Read the model definition and answer for the solid it produces. Units are mm, in the model's axes. Give positions to 0.01 mm unless a question says otherwise; leave off trailing zeros. Order: outer loops, then holes, each group sorted by start corner. A loop starts at its lowest first (then second) coordinate and runs counter-clockwise, first axis right, second up. Notation, with made-up numbers: (-1.5, 61.25) -> (38.5, 61.25) arc R17 cw to (38.5, 67.25) -> close; hole circle Ø7 at (-33.75, 81). An arc over 180 degrees is marked (long way). Use one line per item in the form item = value.
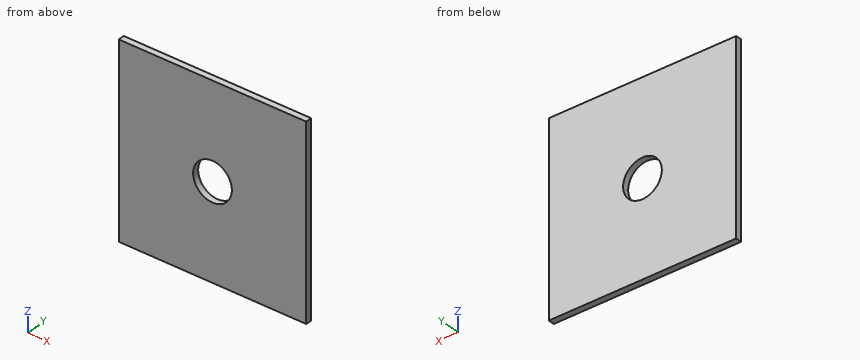
```python
from build123d import *

# Parameters (mm, degrees)
SKETCH2_W                = 30
SKETCH2_H                = 30
BOSS_EXTRUDE1_DEPTH      = 10
SKETCH3_W                = 30
SKETCH3_H                = 30
SKETCH3_W_2              = 25
SKETCH3_H_2              = 25
BOSS_EXTRUDE2_DEPTH      = 15
SKETCH4_W                = 30
SKETCH4_H                = 30
BOSS_EXTRUDE3_DEPTH      = 15
CUT_EXTRUDE1_START       = -40
SKETCH5_R                = 3.05
CUT_EXTRUDE1_DEPTH       = 40
BOSS_EXTRUDE4_DEPTH      = 10
BOSS_EXTRUDE4_DEPTH_BACK = 40
SKETCH6_W                = 7.5
SKETCH6_H                = 1.017843133
SKETCH6_H_2              = 1.2761833
SKETCH7_R                = 2.76
CUT_EXTRUDE2_DEPTH       = 10
SKETCH8_W                = 30
SKETCH8_H                = 30
BOSS_EXTRUDE5_DEPTH      = 1
SKETCH9_R                = 3.1
CUT_EXTRUDE3_DEPTH       = 1


with BuildPart() as part:
    # Sketch2 → Boss-Extrude1 (new body)
    with BuildSketch(Plane(origin=(0, 0, 0), x_dir=(1, 0, 0), z_dir=(0, 1, 0))):
        Rectangle(SKETCH2_W, SKETCH2_H)
    extrude(amount=BOSS_EXTRUDE1_DEPTH)


with BuildPart() as body_2:
    # Sketch3 → Boss-Extrude2 (new body)
    with BuildSketch(Plane(origin=(0, 10, 0), x_dir=(1, 0, 0), z_dir=(0, 1, 0))):
        Rectangle(SKETCH3_W, SKETCH3_H)
        Rectangle(SKETCH3_W_2, SKETCH3_H_2, mode=Mode.SUBTRACT)
    extrude(amount=BOSS_EXTRUDE2_DEPTH)


with BuildPart() as body_3:
    # Sketch4 → Boss-Extrude3 (new body)
    with BuildSketch(Plane(origin=(0, 25, 0), x_dir=(1, 0, 0), z_dir=(0, 1, 0))):
        Rectangle(SKETCH4_W, SKETCH4_H)
    extrude(amount=BOSS_EXTRUDE3_DEPTH)


with BuildPart() as cut_extrude1_tool:
    # Sketch5 → Cut-Extrude1 (new body)
    with BuildSketch(Plane(origin=(0, 40, 0), x_dir=(1, 0, 0), z_dir=(0, 1, 0)).offset(CUT_EXTRUDE1_START)):
        with Locations(Location((0, 0, 0), (0, 0, 270))):
            Circle(SKETCH5_R)
    extrude(amount=CUT_EXTRUDE1_DEPTH)


with BuildPart() as part_1:
    add(part.part)

    # Cut-Extrude1: cut by cut_extrude1_tool
    add(cut_extrude1_tool.part, mode=Mode.SUBTRACT)


with BuildPart() as body_3_1:
    add(body_3.part)

    # Cut-Extrude1: cut by cut_extrude1_tool
    add(cut_extrude1_tool.part, mode=Mode.SUBTRACT)

    # Sketch6 → Boss-Extrude4 (add, two sides: drawn at the far end of the back side and taken through both)
    with BuildSketch(Plane(origin=(0, 0, -15), x_dir=(-1, 0, 0), z_dir=(0, 0, -1)).offset(-BOSS_EXTRUDE4_DEPTH_BACK)):
        with Locations((-11.25, 25.508921566)):
            Rectangle(SKETCH6_W, SKETCH6_H)
        with Locations((11.25, 25.63809165)):
            Rectangle(SKETCH6_W, SKETCH6_H_2)
    extrude(amount=BOSS_EXTRUDE4_DEPTH + BOSS_EXTRUDE4_DEPTH_BACK)

    # Sketch7 → Cut-Extrude2 (cut)
    with BuildSketch(Plane(origin=(0, 26.2761833, 0), x_dir=(1, 0, 0), z_dir=(0, 1, 0))):
        with Locations(Location((-11.25, 20, 0), (0, 0, 270))):
            Circle(SKETCH7_R)
        with Locations(Location((11.25, 20, 0), (0, 0, 270))):
            Circle(SKETCH7_R)
        with Locations(Location((11.25, -20.5, 0), (0, 0, 270))):
            Circle(SKETCH7_R)
        with Locations(Location((-11.25, -20.5, 0), (0, 0, 270))):
            Circle(SKETCH7_R)
    extrude(amount=-CUT_EXTRUDE2_DEPTH, mode=Mode.SUBTRACT)


with BuildPart() as body_2_2:
    # Sketch8 → Boss-Extrude5 (new body)
    with BuildSketch(Plane(origin=(0, 40, 0), x_dir=(1, 0, 0), z_dir=(0, 1, 0))):
        Rectangle(SKETCH8_W, SKETCH8_H)
    extrude(amount=BOSS_EXTRUDE5_DEPTH)

    # Sketch9 → Cut-Extrude3 (cut)
    with BuildSketch(Plane(origin=(0, 41, 0), x_dir=(1, 0, 0), z_dir=(0, 1, 0))):
        with Locations(Location((0, 0, 0), (0, 0, 270))):
            Circle(SKETCH9_R)
    extrude(amount=-CUT_EXTRUDE3_DEPTH, mode=Mode.SUBTRACT)


solid = body_2_2.part
```
Item 1: The part is cut by section C-C on y = 40.8. Give the vertices of the cut face in (x, z).
Checks:
outline = (-15, -15) -> (15, -15) -> (15, 15) -> (-15, 15) -> close; hole circle Ø6.2 at (0, 0)
Item 2: A straight line is drawn through the part: L1, parallel to X at y = 40.65, z = 0. Find the intervals that lie inside material, in ascending order. Write a range as from..to.
Checks:
L1 = -15..-3.1, 3.1..15
Item 3: The part is cut by section B-B on z = 0. Give the vertices of the cut face in (x, y).
Checks:
outline = (-15, 40) -> (-3.1, 40) -> (-3.1, 41) -> (-15, 41) -> close; (3.1, 40) -> (15, 40) -> (15, 41) -> (3.1, 41) -> close
Item 4: The part is cut by section A-A on x = 0. Give the vertices of the cut face in (y, z), and give its area (3 significant figures).
Checks:
outline = (40, -15) -> (41, -15) -> (41, -3.1) -> (40, -3.1) -> close; (40, 3.1) -> (41, 3.1) -> (41, 15) -> (40, 15) -> close
area = 23.8 mm²
